Source: three-view drawing plus pictorial views. Frame: mm from the lowest corner of the part. Give positions to 0.01 mm unless a question says otherwise; leave off trailing zeros. Order: outer loops, then holes, each group sorted by start corner. A loop starts at its lowest first (then second) coordinate and runs counter-clockwise, first axis right, second up. Notation, with made-up numbers: (49, 16) - (97, 16) arc R23 cw to (97, 27) - close; hole circle Ø5 at (-1.5, -0.75). An arc over 180 degrees is marked (long way). Use one line per item in the form item = value.
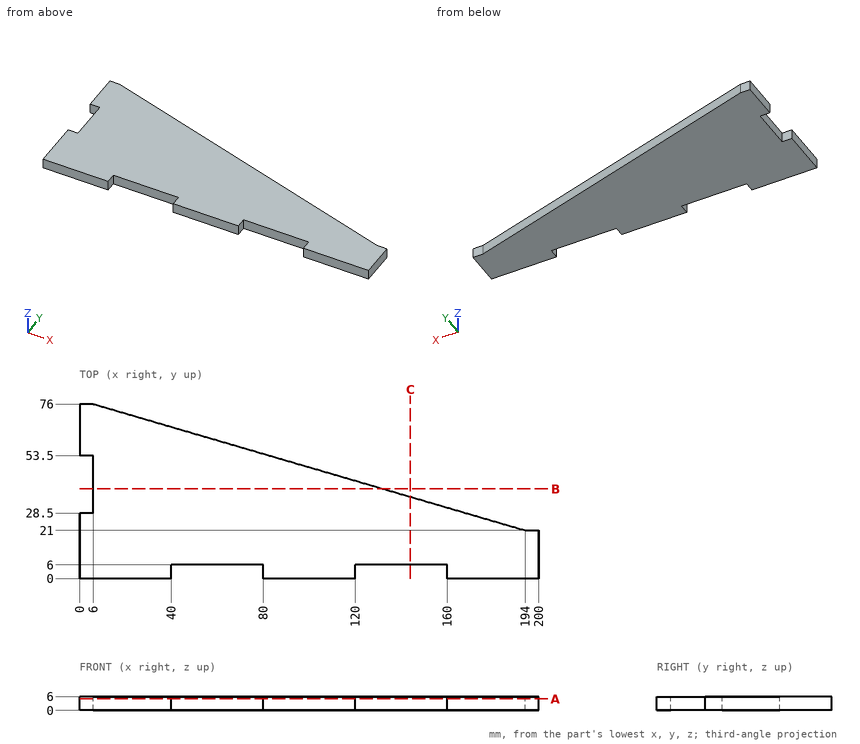
(1) Contact query for flat-ended pins moving along their axis: pin 1 Ø1 at (x, y) = (92, 21) entering from -Z; pin 2 Ø3 at (x, y) = (174, 28.5) entering from -Z; pin 3 Ø3 at (y, z) = (33, 3.5) entering from -X. Output: stop coordinate, or through.
Computed values:
pin_1 = 0
pin_2 = through
pin_3 = 6
(2) Cut plane C-C on x = 144. Output: boundary loops of the cut face in (y, z).
Computed values:
outline = (6, 0) - (35.63, 0) - (35.63, 6) - (6, 6) - close
(3) Ray query, line 1 along X through (y, z) = (4, 3.85); line 2 along Y through (x, z) = (58, 3.15); line 3 along Y through (x, z) = (69, 4.85). Return the intervals inside material, ascending.
Computed values:
line_1 = 0 to 40, 80 to 120, 160 to 200
line_2 = 6 to 60.79
line_3 = 6 to 57.57
(4) Cut plane A-A on z = 5.05. Output: boundary loops of the cut face in (x, y), plus the area to 3 significant figures.
Computed values:
outline = (0, 0) - (40, 0) - (40, 6) - (80, 6) - (80, 0) - (120, 0) - (120, 6) - (160, 6) - (160, 0) - (200, 0) - (200, 21) - (194, 21) - (6, 76) - (0, 76) - (0, 53.5) - (6, 53.5) - (6, 28.5) - (0, 28.5) - close
area = 9,070 mm²
(5) Cut plane B-B on y = 39. Output: boundary loops of the cut face in (x, z).
Computed values:
outline = (6, 0) - (132.47, 0) - (132.47, 6) - (6, 6) - close
